```python
from build123d import *

# Parameters (mm, degrees)
BOX001_W       = 10
BOX001_H       = 10
BOX001_DEPTH   = 8
CYLINDER_R     = 3
CYLINDER_DEPTH = 10
BOX_W          = 16
BOX_H          = 16
BOX_DEPTH      = 10


with BuildPart() as cube001:
    # Box001 → Box001 (new body)
    with BuildSketch(Plane(origin=(-5, -5, 0), x_dir=(1, 0, 0), z_dir=(0, 0, 1))):
        with Locations((5, 5)):
            Rectangle(BOX001_W, BOX001_H)
    extrude(amount=BOX001_DEPTH)


with BuildPart() as cylinder:
    # Cylinder → Cylinder (new body)
    with BuildSketch(Plane.XY.offset(10)):
        Circle(CYLINDER_R)
    extrude(amount=CYLINDER_DEPTH)


with BuildPart() as cut:
    # Box → Box (new body)
    with BuildSketch(Plane(origin=(-8, -8, 0), x_dir=(1, 0, 0), z_dir=(0, 0, 1))):
        with Locations((8, 8)):
            Rectangle(BOX_W, BOX_H)
    extrude(amount=BOX_DEPTH)

    # Fusion: union Cylinder
    add(cylinder.part)

    # Cut: cut Cube001
    add(cube001.part, mode=Mode.SUBTRACT)


solid = cut.part
```
The model under review builds one solid part; all positions refer to its coordinate system, in mm. A direction names the side the tool comes from. Give positions to 0.01 mm unless a question says otherwise; leave off trailing zeros. Write each loop counter-clockwise with the first axis right and the second up, starting at its lowest first coordinate (ties: lowest second). Pieces come first, ordered by that corner, then holes. Notation, with made-up numbers: M -22,-3 L 19,-3 A15 cw 19,7 Z; hole C 48.5,76 d2. An arc over 180 degrees is marked long. Write each question's results on one line, items separated by ' | '. Start each with the question number.
1. We need section B-B (y = 4). Write out the cut boundary in (x, z).
2. Insertion check: pin 1 Ø3 at (x, y) = (0, 1.5) entering from -Z; pin 2 Ø3 at (y, z) = (0.5, 13) entering from +X; pin 3 Ø5 at (x, z) = (-2.5, 14) entering from -Y. Each pin has a flat end and moves straight along its axis. Give the tip position at first contact, or say it passes through.
3. For probe 1 along Y at (x, z) = (0.75, 6.25); probe 2 along Z at (x, y) = (-6.75, 6.25), list the stretches that pass through material, from the lowest coordinate up. Write a range as [from, to].
4. We need section A-A (z = 7.25). Write out the cut boundary in (x, y).
5. We need section C-C (x = 0). Write out the cut boundary in (y, z), and give its area (3 significant figures).
6. Mouldability with a two-part tool opening along Y and no side actions: class faces 4 (the flat face through (-8, 0, 5)), 5 (the flat face through (0, 5, 4)), 6 (the flat face through (0, -8, 5)) as released by +Y, released by -Y, zero draft, split by the parting line, or undercut.
7. For faces 1 (the flat face through (-4, 0, 10)), 2 (the flat face through (0, 0, 20)), 3 (the flat face through (0, -5, 4)), list the 3-axis set-ups (+Z, -Z, +X, -X, +Y, -Y) from which the entire face can be reached by the end or side of a thin tool; tool diameter is ignored.
8. We need section D-D (z = 10.25). Write out the cut boundary in (x, y).
Results found:
1) outline: M -8,0 L -5,0 L -5,8 L 5,8 L 5,0 L 8,0 L 8,10 L -8,10 Z
2) pin 1: stops at z = 8 | pin 2: stops at x = 3 | pin 3: stops at y = -3
3) probe 1: y = [-8, -5], [5, 8] | probe 2: z = [0, 10]
4) outline: M -8,-8 L 8,-8 L 8,8 L -8,8 Z; hole M -5,-5 L 5,-5 L 5,5 L -5,5 Z
5) outline: M -8,0 L -5,0 L -5,8 L 5,8 L 5,0 L 8,0 L 8,10 L 3,10 L 3,20 L -3,20 L -3,10 L -8,10 Z | area: 140 mm^2
6) face 4: zero draft | face 5: undercut | face 6: released by -Y
7) face 1: +Z | face 2: +Z, +X, -X, +Y, -Y | face 3: -Z
8) outline: C 0,0 d6
